Check sheet for the drawn part. Datum: minimum x, y, z corner. Units: mm. Coordinates: 2 decimals unless noted, no trailing zeros. Loops run counter-clockwise (first coordinate to the right, second up) from the corner with the lowest first, then second, coordinate; pieces in that order, holes last.
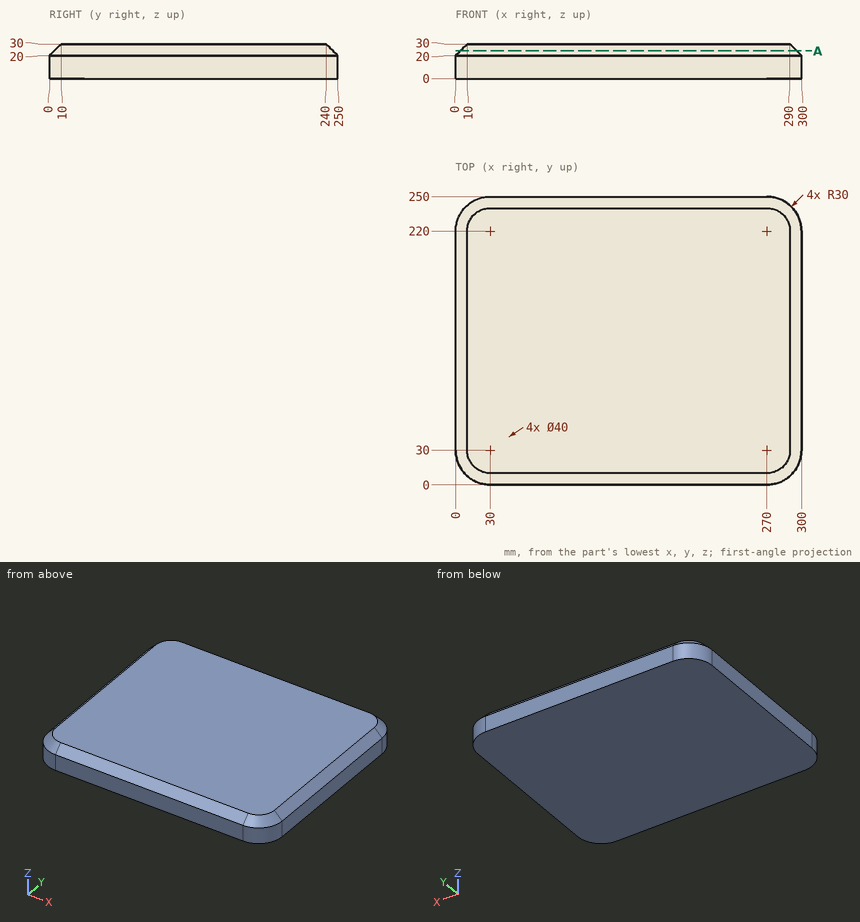
1) Scan lines: line 1 (Y direction, x = 271, z = 6.25); line 2 (X direction, y = 28, z = 7.5); line 3 (X direction, y = 61, z = 26.25). Record each from-to range of solid material in increasing order.
Answer sheet:
line 1: y = 0.02 to 249.98
line 2: x = 0.07 to 299.93
line 3: x = 6.25 to 293.75
2) Depth check by flat-ended pin: pin 1 (10 mm diameter, centred on x = 103, z = 21.5, fed in from -Y); pin 2 (4 mm diameter, centred on x = 246.5, z = 23, fed in from -Y). Enter the tip coordinate at first touch or a pass-through.
Answer sheet:
pin 1: stops at y = 0
pin 2: stops at y = 1
3) Section check A-A on z = 24. Enter the section's corners in (x, y), plus the area to 3 significant figures.
Answer sheet:
outline: (4, 30) arc R26 ccw to (30, 4) - (270, 4) arc R26 ccw to (296, 30) - (296, 220) arc R26 ccw to (270, 246) - (30, 246) arc R26 ccw to (4, 220) - close
area: 70,100 mm2
